CAD build for the part. Positions are in the model's coordinates, mm. A direction names the side the tool comes from. Round coordinates to 2 decimals unless told otherwise and drop trailing zeros. Loops run counter-clockwise (first coordinate to the right, second up) from the corner with the lowest first, then second, coordinate; pieces in that order, holes last. Notation, with made-up numbers: (8, 4) -> (42, 4) arc R22 ccw to (42, 11) -> close; hole circle Ø5 at (-15, 14.5). An arc over 180 degrees is marked (long way). Answer as CSV lines item,"result".
Autodesk Inventor part; units mm, degrees
ref_plane "YZ Plane" through (0, 0, 0) normal (1, 0, 0) x (0, 1, 0)
ref_plane "XZ Plane" through (0, 0, 0) normal (0, 1, 0) x (-1, 0, 0)
ref_plane "XY Plane" through (0, 0, 0) normal (0, 0, 1) x (1, 0, 0)
sketch "Sketch1" plane through (0, 0, 0) normal (0, 1, 0) x (-1, 0, 0)
  line L0 (0, 0) -> (38.1, 0)
  line L1 (38.1, 0) -> (38.1, -19.05)
  line L2 (38.1, -19.05) -> (0, -19.05)
  line L3 (0, -19.05) -> (0, 0)
  circle A0 centre (6.35, -3.175) radius 2.4765
  circle A1 centre (31.75, -3.175) radius 2.4765
  dimension "d0" = 4.953
  dimension "d1" = 4.953
  dimension "d2" = 25.4
  dimension "d3" = 6.35
  dimension "d4" = 3.175
  dimension "d5" = 6.35
  dimension "d6" = 19.05
extrude "Extrusion1" add sketch "Sketch1" along normal blind 6.35
sketch "Sketch2" plane through (0, 0, -19.05) normal (0, 0, -1) x (-1, 0, 0)
  line L0 (38.1, 0) -> (0, 0)
  line L1 (38.1, 0) -> (38.1, 6.35)
  line L2 (0, 6.35) -> (38.1, 6.35)
  line L3 (0, 0) -> (0, 6.35)
  circle A0 centre (19.05, 17.7546) radius 14.2748
  circle A1 centre (19.05, 17.7546) radius 6.35
  line L4 (38.1, 6.35) -> (0, 6.35)
  line L5 (0, 6.35) -> (7.4663, 22.9612)
  line L6 (38.1, 6.35) -> (30.6337, 22.9612)
  arc A2 (30.6337, 22.9612) -> (7.4663, 22.9612) centre (19.05, 17.7546) ccw
  point P0 (0, 0)
  dimension "d9" = 6.35
  dimension "d10" = 12.7
extrude "Extrusion2" add sketch "Sketch2" against normal blind 6.35 contours L2 A0 L6 | L5 A0 L2 | L2 A0 L5 A2 L6
equation "\"d5\" = d3"
properties part number "Encoder mount"
Q1. Probe L1, parallel to Y at x = -19.05, z = -16.75; L2, parallel to X at y = 3.5, z = -1.5; L3, parallel to Z at x = -31.75, y = 1.75. List the from-to ranges inside material, lowest first. Write a range as [from, to].
Results:
L1,"[0, 11.4], [24.1, 30.45]"
L2,"[-38.1, -33.57], [-29.93, -8.17], [-4.53, 0]"
L3,"[-19.05, -5.65], [-0.7, 0]"
Q2. Slice it at C-C, the plane y = 16. Give the cut face in (x, z).
Results:
outline,"(-33.76, -19.05) -> (-25.15, -19.05) -> (-25.15, -12.7) -> (-33.76, -12.7) -> close; (-12.95, -19.05) -> (-4.34, -19.05) -> (-4.34, -12.7) -> (-12.95, -12.7) -> close"
Q3. Slice it at B-B, the plane z = -13.5. Give the cut face in (x, y), and give its area (3 significant figures).
Results:
outline,"(-38.1, 0) -> (0, 0) -> (0, 6.35) -> (-7.47, 22.96) arc R12.7 ccw to (-30.63, 22.96) -> (-38.1, 6.35) -> close; hole circle Ø12.7 at (-19.05, 17.75)"
area,"749 mm2"
Q4. Drop flat-ended pins along their axis: pin 1 Ø2 at (x, z) = (-27.5, -14) entering from +Y; pin 2 Ø8 at (x, y) = (-14.5, 24) entering from +Z; pin 3 Ø1 at (x, z) = (-17.5, -3.5) entering from +Y. Give the stop position or say it passes through.
Results:
pin 1,"y = 28.04"
pin 2,"z = -12.7"
pin 3,"y = 6.35"
Q5. Two-plate mould, pull along X, no slides. Class faces 3 (the flat face through (-3.68, 14.54, -15.92)), 4 (the cylindrical face through (-31.43, 3.13, -5.63)), 5 (the flat face through (-34.42, 14.54, -15.92)): pulls with the +X half, pulls with the -X half, needs draft (parallel to the pull), parting line crosses it, or undercut.
Results:
face 3,"pulls with the +X half"
face 4,"undercut"
face 5,"pulls with the -X half"
Q6. Slice it at A-A, the plane x = -19.05. Give the cut face in (y, z), and give its area (3 significant figures).
Results:
outline,"(0, -19.05) -> (11.4, -19.05) -> (11.4, -12.7) -> (6.35, -12.7) -> (6.35, 0) -> (0, 0) -> close; (24.1, -19.05) -> (30.45, -19.05) -> (30.45, -12.7) -> (24.1, -12.7) -> close"
area,"193 mm2"
Q7. Tool access for faces 1 (the flat face through (-19, 11, -12.7)), 2 (the cylindrical face through (-6.03, 3.13, -5.63)): list every direction of +Z, -Z, +X, -X, +Y, -Y with a clear straight run to the whole face (end or side of a thin tool).
Results:
face 1,"+Z, +X, -X, +Y"
face 2,"+Y, -Y"
Q8. Slice it at D-D, the plane x = -31.75. Give the cut face in (y, z), and give its area (3 significant figures).
Results:
outline,"(0, -19.05) -> (20.48, -19.05) -> (20.48, -12.7) -> (6.35, -12.7) -> (6.35, -5.65) -> (0, -5.65) -> close; (0, -0.7) -> (6.35, -0.7) -> (6.35, 0) -> (0, 0) -> close"
area,"179 mm2"
